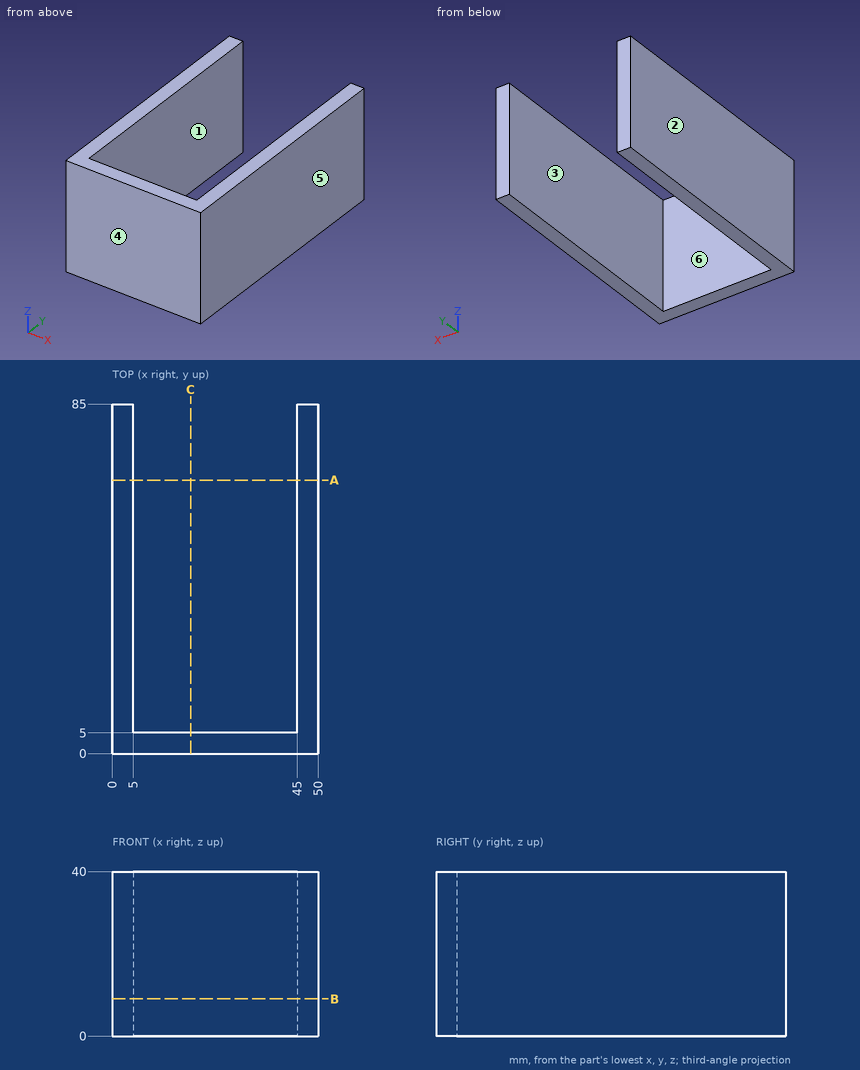
Can you work these out from the drawing? Everything is in mm from the part's minimum corner. A direction names the side the tool comes from. Give positions to 0.01 mm unless a question says otherwise; leave off trailing zeros. Order: outer loops, then holes, each group sorted by start corner. A loop starts at its lowest first (then second) coordinate and runs counter-clockwise, first axis right, second up. Notation, with made-up numbers: (45, 14) -> (59, 14) arc R27 cw to (59, 45) -> close; hole circle Ø3 at (-14.75, -27). An arc over 180 degrees is marked (long way). Return JSON: item names as keys, results as strings.
1. For pin 1 Ø12 at (x, z) = (17.5, 14) entering from +Y, with a flat end and sliding along its axis, tell me the tip position at first contact or that it passes through.
Answer list:
{"pin 1": "stops at y = 5"}
2. Thinking about a two-plate mould opening in X: for the marked faces 3, 4, 5 and 6, which applies, pulls with the +X half, pulls with the -X half, needs draft (parallel to the pull), parting line crosses it, or undercut?
Answer list:
{"face 3": "undercut", "face 4": "needs draft", "face 5": "pulls with the +X half", "face 6": "undercut"}
3. Imagine slicing it at A-A on y = 66.5. List the corners of the cut face in (x, z) for me, then the cut area to 3 significant figures.
Answer list:
{"outline": "(0, 0) -> (5, 0) -> (5, 40) -> (0, 40) -> close; (45, 0) -> (50, 0) -> (50, 40) -> (45, 40) -> close", "area": "400 mm2"}
4. On a 3-axis mill with a long thin cutter (end or side, diameter ignored), from which of +Z, -Z, +X, -X, +Y, -Y can I reach the whole of each face in a straight line? I mean the marked faces 1 and 2. Say none if no direction works.
Answer list:
{"face 1": "+Z, -Z, +Y", "face 2": "+Z, -Z, -X, +Y, -Y"}
5. Imagine slicing it at C-C on x = 19. List the corners of the cut face in (y, z) for me, then the cut area to 3 significant figures.
Answer list:
{"outline": "(0, 0) -> (5, 0) -> (5, 40) -> (0, 40) -> close", "area": "200 mm2"}
6. I need wall thicknesses on line 1 (X direction, y = 79, z = 25.5); line 2 (Y direction, x = 6, z = 18). Which ranges of each line are inside material? Lowest first, please. Write a range as from..to.
Answer list:
{"line 1": "x = 0..5, 45..50", "line 2": "y = 0..5"}
7. Imagine slicing it at B-B on z = 9. List the corners of the cut face in (x, y) for me, then the cut area to 3 significant figures.
Answer list:
{"outline": "(0, 0) -> (50, 0) -> (50, 85) -> (45, 85) -> (45, 5) -> (5, 5) -> (5, 85) -> (0, 85) -> close", "area": "1,050 mm2"}
